```python
from build123d import *

# Parameters (mm, degrees)
CROQUIS1_R              = 2.75
SALIENTE_EXTRUIR1_DEPTH = 10
CROQUIS2_R              = 5
CORTAR_EXTRUIR1_DEPTH   = 2
REDONDEO1_R             = 30


with BuildPart() as part:
    # Croquis1 → Saliente-Extruir1 (new body)
    with BuildSketch(Plane(origin=(0, 0, 0), x_dir=(1, 0, 0), z_dir=(0, 1, 0))):
        Polygon((-148.723962655, -344.2), (-198.723962655, -344.2), (-223.723962655, -300.898729811), (-173.723962655, -300.898729811), align=None)
        with Locations((-173.50486289, -326.5)):
            Circle(CROQUIS1_R, mode=Mode.SUBTRACT)
        with Locations((-196.00486289, -313.509618943)):
            Circle(CROQUIS1_R, mode=Mode.SUBTRACT)
    extrude(amount=SALIENTE_EXTRUIR1_DEPTH)

    # Croquis2 → Cortar-Extruir1 (cut)
    with BuildSketch(Plane(origin=(0, 10, 0), x_dir=(1, 0, 0), z_dir=(0, 1, 0))):
        with Locations((-196.00486289, -313.509618943)):
            Circle(CROQUIS2_R)
        with Locations((-173.50486289, -326.5)):
            Circle(CROQUIS2_R)
    extrude(amount=-CORTAR_EXTRUIR1_DEPTH, mode=Mode.SUBTRACT)

    # Redondeo1
    redondeo1_edges = [part.edges().sort_by_distance(p)[0] for p in [
        (-198.723962655, 5, 344.2),
    ]]
    fillet(redondeo1_edges, radius=REDONDEO1_R)


solid = part.part
```
Verification items for the finished model (mm, model axes). A direction names the side the tool comes from. Coordinates: 2 decimals unless noted, no trailing zeros. Write each loop counter-clockwise with the first axis right and the second up, starting at its lowest first coordinate (ties: lowest second). Pieces come first, ordered by that corner, then holes. Notation, with made-up numbers: (16, 31) - (32, 31) arc R20 ccw to (32, 57) - close; hole circle Ø3 at (35.25, -35.75). An arc over 180 degrees is marked (long way). One line per question, with ' | ' between items. Start each with the question number.
1. Access from +Z, -Z, +X, -X, +Y, -Y to the whole of each face (thin tool, end or side, straight path). Record for faces 1 (the cylindrical face through (-193.32, 9.01, 309.29)), 2 (the cylindrical face through (-196.21, 5.07, 340.29)).
2. Draft check along X on faces 3 (the flat face through (-215.44, 4.93, 315.25)), 4 (the flat face through (-186, 10, 322)), 5 (the cylindrical face through (-194.53, 3.94, 311.19)), 6 (the flat face through (-171, 8, 329)). Enter one of: released by +X, released by -X, zero draft, split by the parting line, or undercut.
3. Gauge pin test, flat ends, axial feed: P1, Ø4, axis at y = 7.5, z = 318.5, coming from the +X side; P2, Ø6.5, axis at x = -196, z = 313.51, coming from the +Y side; P3, Ø1, axis at x = -167, y = 2, coming from the -Z side. Record the tip position at first contact, or that the pin passes through.
4. Material ranges on line 1 along X through (y, z) = (3, 314.5); line 2 along X through (y, z) = (9.3, 326.5); line 3 along Z through (x, y) = (-157, 8.75), recorded low to high.
5. Section check D-D (z = 315.5). Enter the section's corners in (x, y), plus the area to 3 significant figures.
6. Section check C-C (x = -156.5). Enter the section's corners in (y, z).
7. Section check A-A (z = 326.5). Enter the section's corners in (x, y), plus the area to 3 significant figures.
8. Section check B-B (y = 5.5). Enter the section's corners in (x, z).
Computed values:
1) face 1: +Y | face 2: +Z, -X, +Y, -Y
2) face 3: released by -X | face 4: zero draft | face 5: undercut | face 6: undercut
3) P1: x = -162.41 | P2: y = 8 | P3: z = 311.68
4) line 1: -215.87 to -198.57, -193.44 to -165.87 | line 2: -208.94 to -178.5, -168.5 to -158.94 | line 3: 329.87 to 344.2
5) outline: (-215.29, 0) - (-197.9, 0) - (-197.9, 8) - (-200.59, 8) - (-200.59, 10) - (-215.29, 10) - close; (-194.11, 0) - (-165.29, 0) - (-165.29, 10) - (-191.42, 10) - (-191.42, 8) - (-194.11, 8) - close | area: 451 mm²
6) outline: (0, 330.73) - (10, 330.73) - (10, 344.2) - (0, 344.2) - close
7) outline: (-208.94, 0) - (-176.25, 0) - (-176.25, 8) - (-178.5, 8) - (-178.5, 10) - (-208.94, 10) - close; (-170.75, 0) - (-158.94, 0) - (-158.94, 10) - (-168.5, 10) - (-168.5, 8) - (-170.75, 8) - close | area: 436 mm²
8) outline: (-223.72, 300.9) - (-173.72, 300.9) - (-148.72, 344.2) - (-181.4, 344.2) arc R30 ccw to (-207.38, 329.2) - close; hole circle Ø5.5 at (-196, 313.51); hole circle Ø5.5 at (-173.5, 326.5)
